```python
from build123d import *

# Parameters (mm, degrees)
BASE_FLANGE1_START    = -18
BASE_FLANGE1_DEPTH    = 36
FILLET1_R             = 2
M5_TAPPED_HOLE1_D     = 4.2
M5_TAPPED_HOLE1_DEPTH = 4


# Read off the part's stored shape, not the designer's step: Base-Flange1
with BuildPart() as part:
    # Base-Flange1 outline → Base-Flange1 (new body)
    with BuildSketch(Plane.XY.offset(BASE_FLANGE1_START)):
        with BuildLine():
            Line((-5, 45), (-25, 45))
            Line((-25, 45), (-25, 41))
            Line((-25, 41), (-5, 41))
            ThreePointArc((-5, 41), (-4.292893219, 40.707106781), (-4, 40))
            Line((-4, 40), (-4, -40))
            ThreePointArc((-4, -40), (-4.292893219, -40.707106781), (-5, -41))
            Line((-5, -41), (-25, -41))
            Line((-25, -41), (-25, -45))
            Line((-25, -45), (-5, -45))
            ThreePointArc((-5, -45), (-1.464466094, -43.535533906), (0, -40))
            Line((0, -40), (0, 40))
            ThreePointArc((0, 40), (-1.464466094, 43.535533906), (-5, 45))
        make_face()
    extrude(amount=BASE_FLANGE1_DEPTH)

    # Fillet1
    fillet1_edges = [part.edges().sort_by_distance(p)[0] for p in [
        (-25, -43, -18),
        (-25, 43, -18),
        (-25, -43, 18),
        (-25, 43, 18),
    ]]
    fillet(fillet1_edges, radius=FILLET1_R)

    # M5 Tapped Hole1
    with Locations(Plane(origin=(0, 45, 0), x_dir=(1, 0, 0), z_dir=(0, 1, 0))):
        with Locations((-14, 0)):
            m5_tapped_hole1 = Hole(M5_TAPPED_HOLE1_D / 2, depth=M5_TAPPED_HOLE1_DEPTH)

    # Mirror1: M5 Tapped Hole1 across plane
    add(m5_tapped_hole1.mirror(Plane.ZX), mode=Mode.SUBTRACT)


solid = part.part
```
Verification items for the finished model (mm, model axes). A direction names the side the tool comes from. Give positions to 0.01 mm unless a question says otherwise; leave off trailing zeros. Loops run counter-clockwise (first coordinate to the right, second up) from the corner with the lowest first, then second, coordinate; pieces in that order, holes last.
1. Section check D-D, the plane z = -4. Enter the section's corners in (x, y).
2. Section check B-B, the plane z = 0. Enter the section's corners in (x, y), then the cut area to 3 significant figures.
3. Set-up check for faces 1 (the flat face through (-2, 10, 18)), 2 (the flat face through (-17, 41, 0)): record each of +Z, -Z, +X, -X, +Y, -Y from which the full face is reachable in a straight line by a thin tool's end or side.
4. Section check C-C, the plane x = -18.25. Enter the section's corners in (y, z).
5. Thickness scan on line 1 (Y direction, x = -11.25, z = 5); line 2 (Z direction, x = -14, y = 43.8); line 3 (X direction, y = -7, z = -9.5). Record the ranges inside material, lowest first.
6. Mould release check, pull along Y, two halves, no side actions. Record for faces 3 (the flat face through (-17, -41, 0)), 4 (the flat face through (-17, -45, 0)), 5 (the cylindrical face through (-1, 43, 0)), 6 (the flat face through (-25, 43, 0)): released by +Y, released by -Y, zero draft, split by the parting line, or undercut.
7. Section check A-A, the plane x = -14. Enter the section's corners in (y, z).
8. Go/stop test with flat-tipped pins: pin 1 Ø8 at (y, z) = (34.5, 6) entering from -X; pin 2 Ø12 at (x, z) = (-3.5, 9) entering from -Y; pin 3 Ø3.5 at (x, z) = (-14, 0) entering from -Y. Record where each tip stops, or that it passes through.
Geometry says:
1. outline: (-25, -45) - (-5, -45) arc R5 ccw to (0, -40) - (0, 40) arc R5 ccw to (-5, 45) - (-25, 45) - (-25, 41) - (-5, 41) arc R1 cw to (-4, 40) - (-4, -40) arc R1 cw to (-5, -41) - (-25, -41) - close
2. outline: (-25, -45) - (-16.1, -45) - (-16.1, -41) - (-25, -41) - close; (-25, 41) - (-16.1, 41) - (-16.1, 45) - (-25, 45) - close; (-11.9, -45) - (-5, -45) arc R5 ccw to (0, -40) - (0, 40) arc R5 ccw to (-5, 45) - (-11.9, 45) - (-11.9, 41) - (-5, 41) arc R1 cw to (-4, 40) - (-4, -40) arc R1 cw to (-5, -41) - (-11.9, -41) - close
2. area: 484 mm2
3. face 1: +Z, +X, -X, +Y, -Y
3. face 2: +Z, -Z, -X
4. outline: (-45, -18) - (-41, -18) - (-41, 18) - (-45, 18) - close; (41, -18) - (45, -18) - (45, 18) - (41, 18) - close
5. line 1: y = -45 to -41, 41 to 45
5. line 2: z = -18 to -2.1, 2.1 to 18
5. line 3: x = -4 to 0
6. face 3: undercut
6. face 4: released by -Y
6. face 5: released by +Y
6. face 6: zero draft
7. outline: (-45, -18) - (-41, -18) - (-41, -2.1) - (-45, -2.1) - close; (-45, 2.1) - (-41, 2.1) - (-41, 18) - (-45, 18) - close; (41, -18) - (45, -18) - (45, -2.1) - (41, -2.1) - close; (41, 2.1) - (45, 2.1) - (45, 18) - (41, 18) - close
8. pin 1: stops at x = -4
8. pin 2: stops at y = -45
8. pin 3: passes through
